from build123d import *

# Parameters (mm, degrees)
BOSS_EXTRUDE1_DEPTH     = 40
CUT_EXTRUDE1_START      = 10
SKETCH2_R               = 2.6
CUT_EXTRUDE1_DEPTH      = 113.46950766
SKETCH9_W               = 50
SKETCH9_H               = 80
BOSS_EXTRUDE2_DEPTH     = 5
SKETCH11_W              = 24
SKETCH11_H              = 45
BOSS_EXTRUDE3_DEPTH     = 10
CUT_EXTRUDE2_DEPTH      = 117.086174887
CUT_EXTRUDE2_DEPTH_BACK = 117.086174887
SKETCH12_R              = 4.1
CUT_EXTRUDE3_START      = 10
SKETCH13_R              = 6.5
CUT_EXTRUDE3_DEPTH      = 5
FILLET2_R               = 5
CHAMFER1_SIZE           = 2
SKETCH14_W              = 98
SKETCH14_H              = 12
BOSS_EXTRUDE4_DEPTH     = 3
CUT_EXTRUDE4_DEPTH      = 117.086174887
CUT_EXTRUDE4_DEPTH_BACK = 117.086174887
SKETCH12_2_R            = 4.1
CHAMFER2_SIZE           = 1


with BuildPart() as part:
    # Sketch1 → Boss-Extrude1 (new body)
    with BuildSketch(Plane.XY):
        Polygon((0, 0), (0, 80), (10, 80), (10, 10), (40, 10), (40, 70), (15, 70), (15, 80), (50, 80), (50, 0), align=None)
    extrude(amount=BOSS_EXTRUDE1_DEPTH)

    # Sketch2 → Cut-Extrude1 (cut, through all)
    with BuildSketch(Plane(origin=(0, 0, 0), x_dir=(0, 0, -1), z_dir=(1, 0, 0)).offset(CUT_EXTRUDE1_START)):
        with Locations(Location((-20, 30, 0), (0, 0, 270))):
            Circle(SKETCH2_R)
    extrude(amount=-CUT_EXTRUDE1_DEPTH, mode=Mode.SUBTRACT)

    # Sketch9 → Boss-Extrude2 (add)
    with BuildSketch(Plane.XY):
        with Locations((25, 40)):
            Rectangle(SKETCH9_W, SKETCH9_H)
    extrude(amount=-BOSS_EXTRUDE2_DEPTH)

    # Sketch11 → Boss-Extrude3 (add)
    with BuildSketch(Plane(origin=(0, 0, 0), x_dir=(1, 0, 0), z_dir=(0, 1, 0))):
        with Locations((62, -17.5)):
            Rectangle(SKETCH11_W, SKETCH11_H)
        with Locations((-12, -17.5)):
            Rectangle(SKETCH11_W, SKETCH11_H)
    extrude(amount=BOSS_EXTRUDE3_DEPTH)

    # Sketch12 → Cut-Extrude2 (cut, two sides: drawn at the far end of the back side and taken through both)
    with BuildSketch(Plane(origin=(0, 0, 0), x_dir=(1, 0, 0), z_dir=(0, 1, 0)).offset(-CUT_EXTRUDE2_DEPTH_BACK)):
        with Locations(Location((-12, -17.5, 0), (0, 0, 90))):
            Circle(SKETCH12_R)
        with Locations(Location((62, -17.5, 0), (0, 0, 90))):
            Circle(SKETCH12_R)
    extrude(amount=CUT_EXTRUDE2_DEPTH + CUT_EXTRUDE2_DEPTH_BACK, mode=Mode.SUBTRACT)

    # Sketch13 → Cut-Extrude3 (cut)
    with BuildSketch(Plane(origin=(0, 0, 0), x_dir=(1, 0, 0), z_dir=(0, 1, 0)).offset(CUT_EXTRUDE3_START)):
        with Locations(Location((-12, -17.5, 0), (0, 0, 90))):
            Circle(SKETCH13_R)
        with Locations(Location((62, -17.5, 0), (0, 0, 90))):
            Circle(SKETCH13_R)
    extrude(amount=-CUT_EXTRUDE3_DEPTH, mode=Mode.SUBTRACT)

    # Fillet2
    fillet2_edges = [part.edges().sort_by_distance(p)[0] for p in [
        (0, 10, 17.5),
        (50, 10, 17.5),
    ]]
    fillet(fillet2_edges, radius=FILLET2_R)

    # Chamfer1
    chamfer1_edges = [part.edges().sort_by_distance(p)[0] for p in [
        (-14.5, 10, 40),
        (51.464466094, 11.464466094, -5),
        (51.464466094, 11.464466094, 40),
        (-1.464466094, 11.464466094, 40),
        (-1.464466094, 11.464466094, -5),
        (32.5, 80, 40),
        (0, 80, 17.5),
        (50, 80, 17.5),
        (25, 80, -5),
        (0, 47.5, -5),
        (5, 80, 40),
        (0, 47.5, 40),
        (-24, 10, 17.5),
        (-14.5, 10, -5),
        (74, 10, 17.5),
        (64.5, 10, 40),
        (50, 47.5, 40),
        (50, 47.5, -5),
        (64.5, 10, -5),
    ]]
    chamfer(chamfer1_edges, length=CHAMFER1_SIZE)

    # Sketch14 → Boss-Extrude4 (add)
    with BuildSketch(Plane(origin=(0, 0, 0), x_dir=(1, 0, 0), z_dir=(0, 1, 0))):
        with Locations((25, -17.5)):
            Rectangle(SKETCH14_W, SKETCH14_H)
    extrude(amount=-BOSS_EXTRUDE4_DEPTH)

    # Sketch12<2> → Cut-Extrude4 (cut, two sides: drawn at the far end of the back side and taken through both)
    with BuildSketch(Plane(origin=(0, 0, 0), x_dir=(1, 0, 0), z_dir=(0, 1, 0)).offset(-CUT_EXTRUDE4_DEPTH_BACK)):
        with Locations(Location((-12, -17.5, 0), (0, 0, 90))):
            Circle(SKETCH12_2_R)
        with Locations(Location((62, -17.5, 0), (0, 0, 90))):
            Circle(SKETCH12_2_R)
    extrude(amount=CUT_EXTRUDE4_DEPTH + CUT_EXTRUDE4_DEPTH_BACK, mode=Mode.SUBTRACT)

    # Chamfer2
    chamfer2_edges = [part.edges().sort_by_distance(p)[0] for p in [
        (25, -3, 11.5),
        (25, -3, 23.5),
    ]]
    chamfer(chamfer2_edges, length=CHAMFER2_SIZE)


solid = part.part
Check sheet for the modelled part. Datum: model origin and axes. Units: mm. A direction names the side the tool comes from. Coordinates: 2 decimals unless noted, no trailing zeros. Loops run counter-clockwise (first coordinate to the right, second up) from the corner with the lowest first, then second, coordinate; pieces in that order, holes last. Notation, with made-up numbers: (16.25, -36) -> (62.25, -36) arc R7 cw to (62.25, -25) -> close; hole circle Ø10 at (37, -5.5). An arc over 180 degrees is marked (long way). Answer in a Markdown table with one row per item.
1. Sectioned sample at C-C, the plane y = 73. Record the boundary of the cut face in (x, z), then the cut area to 3 significant figures.
Check values:
| item | result |
|---|---|
| outline | (0, -3) -> (2, -5) -> (48, -5) -> (50, -3) -> (50, 38) -> (48, 40) -> (15, 40) -> (15, 0) -> (10, 0) -> (10, 40) -> (2, 40) -> (0, 38) -> close |
| area | 2,040 mm2 |
2. Go/stop test with flat-tipped pins: pin 1 (4 mm diameter, centred on x = -15, z = 14.5, fed in from +Y); pin 2 (1 mm diameter, centred on x = 50, z = 31, fed in from -Y); pin 3 (12 mm diameter, centred on y = 45.5, z = 14, fed in from -X). Record where each tip stops, or that it passes through.
Check values:
| item | result |
|---|---|
| pin 1 | stops at y = 5 |
| pin 2 | stops at y = 0 |
| pin 3 | stops at x = 0 |
3. Sectioned sample at B-B, the plane x = -12. Record the boundary of the cut face in (y, z).
Check values:
| item | result |
|---|---|
| outline | (-3, 12.5) -> (-2, 11.5) -> (0, 11.5) -> (0, -5) -> (8, -5) -> (10, -3) -> (10, 11) -> (5, 11) -> (5, 13.4) -> (-3, 13.4) -> close; (-3, 21.6) -> (5, 21.6) -> (5, 24) -> (10, 24) -> (10, 38) -> (8, 40) -> (0, 40) -> (0, 23.5) -> (-2, 23.5) -> (-3, 22.5) -> close |
4. Release check for a two-part mould opening along Y. For faces 4 (the face through (28, 70, 20)), 5 (the face through (24, -3, 17)), 6 (the face through (43, 30, 40)), 7 (the face through (-2, 11, 17)) record: released by +Y, released by -Y, zero draft, split by the parting line, or undercut.
Check values:
| item | result |
|---|---|
| face 4 | undercut |
| face 5 | released by -Y |
| face 6 | zero draft |
| face 7 | released by +Y |
5. Access from +Z, -Z, +X, -X, +Y, -Y to the whole of each face (thin tool, end or side, straight path). Record for faces 1 (the face through (62, 5, 13)), 2 (the face through (50, 46, 18)), 3 (the face through (-19, 10, 17)).
Check values:
| item | result |
|---|---|
| face 1 | +Y |
| face 2 | +Z, -Z, +X, +Y |
| face 3 | +Z, -Z, -X, +Y |
6. Material ranges on line 1 along X through (y, z) = (0.5, 17.5); line 2 along X through (y, z) = (49.5, 26); line 3 along Z through (x, y) = (2.5, 30), recorded low to high. Write a range as [from, to].
Check values:
| item | result |
|---|---|
| line 1 | x = [-24, -16.1], [-7.9, 57.9], [66.1, 74] |
| line 2 | x = [0, 10], [40, 50] |
| line 3 | z = [-5, 17.4], [22.6, 40] |
7. Sectioned sample at D-D, the plane z = 9. Record the boundary of the cut face in (x, y), then the cut area to 3 significant figures.
Check values:
| item | result |
|---|---|
| outline | (-24, 0) -> (74, 0) -> (74, 8) -> (72, 10) -> (55, 10) arc R5 cw to (50, 15) -> (50, 78) -> (48, 80) -> (15, 80) -> (15, 70) -> (40, 70) -> (40, 10) -> (10, 10) -> (10, 80) -> (2, 80) -> (0, 78) -> (0, 15) arc R5 cw to (-5, 10) -> (-22, 10) -> (-24, 8) -> close |
| area | 2,630 mm2 |
8. Sectioned sample at A-A, the plane y = 30. Record the boundary of the cut face in (x, z).
Check values:
| item | result |
|---|---|
| outline | (0, -3) -> (2, -5) -> (48, -5) -> (50, -3) -> (50, 38) -> (48, 40) -> (40, 40) -> (40, 0) -> (10, 0) -> (10, 17.4) -> (0, 17.4) -> close; (0, 22.6) -> (10, 22.6) -> (10, 40) -> (2, 40) -> (0, 38) -> close |
